Design review of the part shown in the three views and the two pictorial views. Dimensions are in mm from the part's minimum x, y and z. Round coordinates to 2 decimals unless told otherwise and drop trailing zeros.
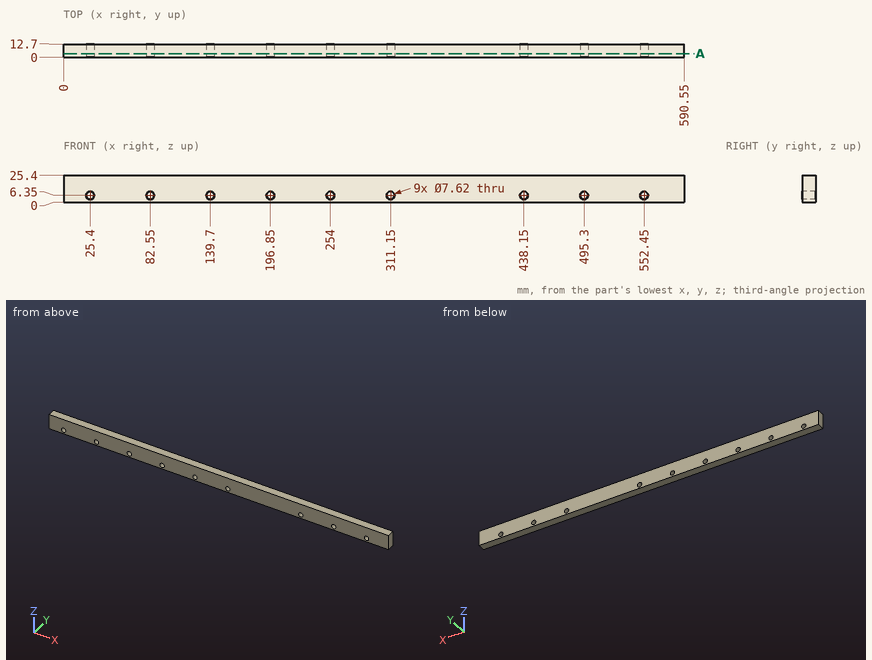
1) Clearance check with a flat-ended pin moving along its axis: P1, Ø6, axis at x = 82.55, z = 6.35, coming from the +Y side. State where the tip first meets the part, or that it passes through.
Results:
P1: passes through
2) To check wall thickness, follow line 1 along Z through (x, y) = (196.85, 5); line 2 along Z through (x, y) = (141, 10). State the ranges of each line that lie inside material, in increasing order.
Results:
line 1: z = 0 to 2.54, 10.16 to 25.4
line 2: z = 0 to 2.77, 9.93 to 25.4
3) Take a section at A-A on y = 3.5. State how many separate pieces and enclosed holes the cut face has, plus the area to 3 significant figures.
Results:
separate pieces: 1
enclosed holes: 9
area: 14,600 mm2
